The listing builds one solid part. Answer for the finished solid, in the listing's coordinates (mm). Face numbers are marked on the shaded views. Coordinates: 2 decimals unless noted, no trailing zeros. Order: outer loops, then holes, each group sorted by start corner. A loop starts at its lowest first (then second) coordinate and runs counter-clockwise, first axis right, second up. Notation, with made-up numbers: (57.25, 64.25) -> (89.25, 64.25) arc R26 cw to (89.25, 100.25) -> close; hole circle Ø3 at (3, 85). An arc over 180 degrees is marked (long way). Return JSON: item names as keys, results as strings.
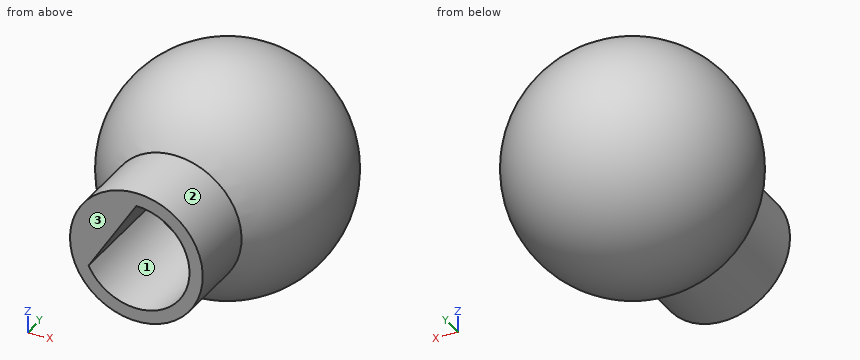
```python
from build123d import *

# Parameters (mm, degrees)
SKETCH_1_R          = 4
EXTRUDE_1_DEPTH     = 10
CUT_EXTRUDE_1_DEPTH = 7


with BuildPart() as part:
    # 草图1 → 凸台-拉伸1 (new body)
    with BuildSketch(Plane(origin=(0, 0, 0), x_dir=(1, 0, 0), z_dir=(0, 1, 0))):
        with Locations(Location((0, 0, 0), (0, 0, 270))):
            Circle(SKETCH_1_R)
    extrude(amount=EXTRUDE_1_DEPTH)

    # 草图2 → 旋转1 (revolve)
    with BuildSketch(Plane(origin=(0, 10, 0), x_dir=(1, 0, 0), z_dir=(0, 1, 0))):
        with BuildLine():
            Line((0, 7), (0, -7))
            ThreePointArc((0, -7), (7, 0), (0, 7))
        make_face()
    revolve(axis=Axis((0, 10, -7), (0, 0, 1)))

    # 草图3 → 切除-拉伸1 (cut)
    with BuildSketch(Plane.XZ):
        with BuildLine():
            Line((0, 3.2), (-2.879179207, -1.396541118))
            ThreePointArc((-2.879179207, -1.396541118), (2.711911833, -1.698686025), (0, 3.2))
        make_face()
    extrude(amount=-CUT_EXTRUDE_1_DEPTH, mode=Mode.SUBTRACT)


solid = part.part
```
Item 1: The part is cut by section C-C on y = 6.5. Determine the outline of the cut face in (x, z).
Answer list:
{"outline": "circle Ø12.12 at (0, 0); hole (-2.88, -1.4) arc R3.2 ccw (long way) to (0, 3.2) -> close"}
Item 2: The part is cut by section D-D on z = 6.25. Determine the outline of the cut face in (x, y), plus the area to 3 significant figures.
Answer list:
{"outline": "circle Ø6.3 at (0, 10)", "area": "31.2 mm2"}
Item 3: Find the intervals of material crossed by probe 1 along X at (y, z) = (2, -2.5); probe 2 along X at (y, z) = (3, 0); probe 3 along Z at (x, y) = (-2, 6.75), in increasing order.
Answer list:
{"probe 1": "-3.12 to -2, 2 to 3.12", "probe 2": "-4 to -2, 3.2 to 4", "probe 3": "-5.87 to -2.5, 0.01 to 5.87"}
Item 4: The part is cut by section B-B on x = 2. Determine the outline of the cut face in (y, z), plus the area to 3 significant figures.
Answer list:
{"outline": "(0, -3.46) -> (4.26, -3.46) arc R6.71 ccw (long way) to (4.26, 3.46) -> (0, 3.46) -> (0, 2.5) -> (7, 2.5) -> (7, -2.5) -> (0, -2.5) -> close", "area": "131 mm2"}
Item 5: Determine the mould class of the marked faces 1, 2 and 3 for opening direction Z: pulls with the +Z half, pulls with the -Z half, needs draft (parallel to the pull), parting line crosses it, or undercut.
Answer list:
{"face 1": "undercut", "face 2": "parting line crosses it", "face 3": "needs draft"}
Item 6: Flat-ended cylindrical pins translate along their axes: pin 1 (2 mm diameter, centred on x = 3, z = -1, fed in from +Y); pin 2 (1 mm diameter, centred on x = 4.5, y = 7.5, fed in from -Z); pin 3 (3 mm diameter, centred on y = 11.5, z = -5.5, fed in from +X); pin 4 (5 mm diameter, centred on x = 0, z = 0, fed in from -Y). Find the tip coordinate at first contact, or state that the pin passes through.
Answer list:
{"pin 1": "y = 16.66", "pin 2": "z = -5.23", "pin 3": "x = 5.6", "pin 4": "y = 0"}
Item 7: The part is cut by section A-A on z = -2. Determine the outline of the cut face in (x, y).
Answer list:
{"outline": "(-3.46, 0) -> (-2.5, 0) -> (-2.5, 7) -> (2.5, 7) -> (2.5, 0) -> (3.46, 0) -> (3.46, 4.26) arc R6.71 ccw (long way) to (-3.46, 4.26) -> close"}
